Design review of the part built by this model. Coordinates are the model's own, in mm. Face numbers are marked on the shaded views. Give positions to 0.01 mm unless a question says otherwise; leave off trailing zeros. Loops run counter-clockwise (first coordinate to the right, second up) from the corner with the lowest first, then second, coordinate; pieces in that order, holes last. Notation, with made-up numbers: (83.5, 48.5) - (138.5, 48.5) arc R25 cw to (138.5, 73.5) - close; hole circle Ø2 at (-23.5, 42). An arc over 180 degrees is marked (long way). Write each question's results on one line, items separated by ' | '.
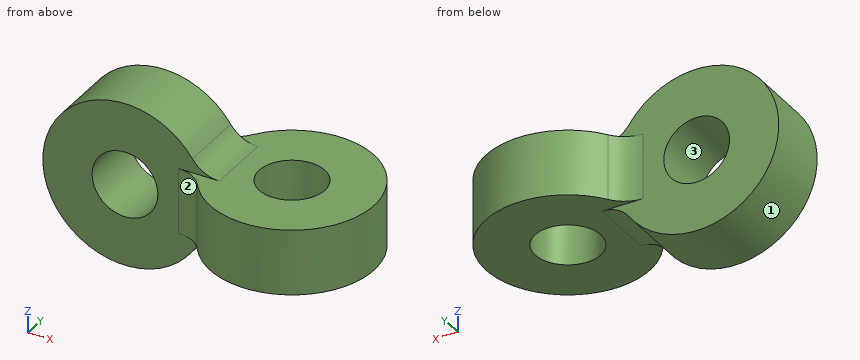
```python
from build123d import *

# Parameters (mm, degrees)
SKETCH1_R           = 2.5
SKETCH1_R_2         = 1
BOSS_EXTRUDE2_DEPTH = 2
SKETCH2_R           = 2.5
SKETCH2_R_2         = 1
BOSS_EXTRUDE3_DEPTH = 1
FILLET3_R           = 1
FILLET4_R           = 1
FILLET5_R           = 1
FILLET8_R           = 1


with BuildPart() as part:
    # Sketch1 → Boss-Extrude2 (new body)
    with BuildSketch(Plane(origin=(0, 0, 0), x_dir=(1, 0, 0), z_dir=(0, 1, 0))):
        with Locations(Location((0, 0, 0), (0, 0, 270))):
            Circle(SKETCH1_R)
        with Locations(Location((0, 0, 0), (0, 0, 270))):
            Circle(SKETCH1_R_2, mode=Mode.SUBTRACT)
    extrude(amount=BOSS_EXTRUDE2_DEPTH)

    # Sketch2 → Boss-Extrude3 (add, symmetric)
    with BuildSketch(Plane.XY):
        with Locations((4.5, 1)):
            Circle(SKETCH2_R)
        with Locations((4.5, 1)):
            Circle(SKETCH2_R_2, mode=Mode.SUBTRACT)
    extrude(amount=BOSS_EXTRUDE3_DEPTH, both=True)

    # Fillet3
    fillet3_edges = [part.edges().sort_by_distance(p)[0] for p in [
        (2.208712153, 2, 0),
    ]]
    fillet(fillet3_edges, radius=FILLET3_R)

    # Fillet4
    fillet4_edges = [part.edges().sort_by_distance(p)[0] for p in [
        (2.208712153, 0, 0),
    ]]
    fillet(fillet4_edges, radius=FILLET4_R)

    # Fillet5
    fillet5_edges = [part.edges().sort_by_distance(p)[0] for p in [
        (2.291287847, 1, -1),
    ]]
    fillet(fillet5_edges, radius=FILLET5_R)

    # Fillet8
    fillet8_edges = [part.edges().sort_by_distance(p)[0] for p in [
        (2.291287847, 1, 1),
    ]]
    fillet(fillet8_edges, radius=FILLET8_R)


solid = part.part
```
Item 1: Clearance check with flat-ended pins moving along their axes: P1, Ø1.5, axis at x = 2.5, z = 0, coming from the +Y side; P2, Ø2.5, axis at x = 5, y = 1, coming from the -Z side; P3, Ø2, axis at x = 3, y = 0.5, coming from the +Z side. State where each tip first meets the part, or that it passes through.
Output values:
P1: stops at y = 3.17 | P2: stops at z = -1 | P3: stops at z = 1.5
Item 2: We need section A-A on y = 1. Give the boundary of the cut face in (x, z).
Output values:
outline: (2.05, -1.43) arc R1 cw to (2.87, -1) - (3.5, -1) - (3.5, 1) - (2.87, 1) arc R1 cw to (2.05, 1.43) arc R2.5 ccw (long way) to start; (5.5, -1) - (7, -1) - (7, 1) - (5.5, 1) - close; hole circle Ø2 at (0, 0)
Item 3: We need section B-B on z = 0. Give the boundary of the cut face in (x, y).
Output values:
outline: (-2.5, 0) - (-1, 0) - (-1, 2) - (-2.5, 2) - close; (1, 0) - (1.63, 0) arc R1 cw to (2.45, -0.43) arc R2.5 ccw (long way) to (2.45, 2.43) arc R1 cw to (1.63, 2) - (1, 2) - close; hole circle Ø2 at (4.5, 1)
Item 4: We need section D-D on x = 2.25. Give the boundary of the cut face in (y, z), then the cut area to 3 significant figures.
Output values:
outline: (-0.22, -1) - (0, -1) - (0, -1.22) - (2, -1.22) - (2, -1) - (2.22, -1) - (2.22, 1) - (2, 1) - (2, 1.22) - (0, 1.22) - (0, 1) - (-0.22, 1) - close | area: 5.74 mm²
Item 5: Draft analysis for pull direction X (two halves, no side actions). For the marked faces 1, 2 and 3, state which applies: +X half, -X half, draft (parallel to the pull), parting line (faces both ways), or undercut.
Output values:
face 1: parting line | face 2: -X half | face 3: undercut
Item 6: Wall thickness on probe 1 along Y at (x, z) = (4.5, -0.1); probe 2 along X at (y, z) = (0.95, 0); probe 3 along X at (y, z) = (1.35, 0): over which ranges is each line inside the solid? List them lowest first.
Output values:
probe 1: y = -1.5 to 0, 2 to 3.5 | probe 2: x = -2.5 to -1, 1 to 3.5, 5.5 to 7 | probe 3: x = -2.5 to -1, 1 to 3.56, 5.44 to 6.98
Item 7: We need section C-C on x = 0. Give the boundary of the cut face in (y, z), then the cut area to 3 significant figures.
Output values:
outline: (0, -2.5) - (2, -2.5) - (2, -1) - (0, -1) - close; (0, 1) - (2, 1) - (2, 2.5) - (0, 2.5) - close | area: 6.00 mm²
